from build123d import *

# Parameters (mm, degrees)
SKETCH1_R               = 17.526
BOSS_EXTRUDE1_DEPTH     = 2.286
CUT_EXTRUDE1_DEPTH      = 25.890704048
CUT_EXTRUDE1_DEPTH_BACK = 25.890704048


with BuildPart() as part:
    # Sketch1 → Boss-Extrude1 (new body)
    with BuildSketch(Plane.XY):
        Circle(SKETCH1_R)
    extrude(amount=BOSS_EXTRUDE1_DEPTH)

    # Sketch2 → Cut-Extrude1 (cut, two sides: drawn at the far end of the back side and taken through both)
    with BuildSketch(Plane(origin=(0, 0, 0), x_dir=(-1, 0, 0), z_dir=(0, 0, -1)).offset(-CUT_EXTRUDE1_DEPTH_BACK)):
        Polygon((3.683, 6.379143124), (-3.683, 6.379143124), (-7.366, 0), (-3.683, -6.379143124), (3.683, -6.379143124), (7.366, 0), align=None)
    extrude(amount=CUT_EXTRUDE1_DEPTH + CUT_EXTRUDE1_DEPTH_BACK, mode=Mode.SUBTRACT)


solid = part.part
Build history of the part. All positions in model axes, mm. A direction names the side the tool comes from. Give positions to 0.01 mm unless a question says otherwise; leave off trailing zeros. Order: outer loops, then holes, each group sorted by start corner. A loop starts at its lowest first (then second) coordinate and runs counter-clockwise, first axis right, second up. Notation, with made-up numbers: M 47.25,71 L 58.25,71 A9 cw 58.25,83 Z; hole C 27,77 d2. An arc over 180 degrees is marked long. Put each result on its own line as item: value.
Item 1: Slice it at D-D, the plane x = 10. Write the cut outline in (y, z).
From the geometry:
outline: M -14.39,0 L 14.39,0 L 14.39,2.29 L -14.39,2.29 Z
Item 2: Probe line 1 (Y direction, x = 0.5, z = 1.3); line 2 (Y direction, x = -6, z = 1.5); line 3 (X direction, y = -4.5, z = 1.5). List the from-to ranges inside material, lowest first. Write a range as [from, to].
From the geometry:
line 1: y = [-17.52, -6.38], [6.38, 17.52]
line 2: y = [-16.47, -2.37], [2.37, 16.47]
line 3: x = [-16.94, -4.77], [4.77, 16.94]
Item 3: Slice it at B-B, the plane z = 1.55. Write the cut outline in (x, y), plus the area to 3 significant figures.
From the geometry:
outline: C 0,0 d35.05; hole M -7.37,0 L -3.68,-6.38 L 3.68,-6.38 L 7.37,0 L 3.68,6.38 L -3.68,6.38 Z
area: 824 mm2
Item 4: Flat gauge pins, fed straight in: pin 1 Ø1 at (y, z) = (10.5, 1.5) entering from -X; pin 2 Ø8 at (x, y) = (-8.5, -2) entering from -Z; pin 3 Ø0.7 at (x, z) = (-2, 1) entering from -Y. Where does each tip first touch, or does it go through?
From the geometry:
pin 1: stops at x = -14.39
pin 2: stops at z = 0
pin 3: stops at y = -17.45
Item 5: Two-plate mould, pull along X, no slides. Class faces 3 (the flat face through (8, 0, 0)), 4 (the cylindrical face through (16.72, 5.26, 1.13)), 5 (the flat face through (5.55, -3.145, 1.159)): +X half, -X half, draft (parallel to the pull), parting line (faces both ways), or undercut.
From the geometry:
face 3: draft
face 4: parting line
face 5: undercut
Item 6: 3-axis set-ups, long thin cutter, end or side, ignore diameter. For faces 1 (the flat face through (-5.55, 3.145, 1.159)), 2 (the flat face through (8, 0, 2.286)): which of +Z, -Z, +X, -X, +Y, -Y reach the whole face in a straight line?
From the geometry:
face 1: +Z, -Z
face 2: +Z, +X, -X, +Y, -Y
Item 7: Slice it at C-C, the plane y = 3.5. Write the cut outline in (x, z).
From the geometry:
outline: M -17.17,0 L -5.35,0 L -5.35,2.29 L -17.17,2.29 Z; M 5.35,0 L 17.17,0 L 17.17,2.29 L 5.35,2.29 Z
Item 8: Slice it at A-A, the plane x = 0. Write the cut outline in (y, z).
From the geometry:
outline: M -17.53,0 L -6.38,0 L -6.38,2.29 L -17.53,2.29 Z; M 6.38,0 L 17.53,0 L 17.53,2.29 L 6.38,2.29 Z
